```python
from build123d import *

# Parameters (mm, degrees)
SKETCH1_R           = 1.5
BOSS_EXTRUDE1_DEPTH = 8
SKETCH2_R           = 4
SKETCH2_R_2         = 1.5
BOSS_EXTRUDE2_DEPTH = 2
SKETCH4_R           = 4
SKETCH4_R_2         = 2.75
BOSS_EXTRUDE3_DEPTH = 2.5
CUT_EXTRUDE1_DEPTH  = 3
BOSS_EXTRUDE4_DEPTH = 5
BOSS_EXTRUDE5_DEPTH = 2.5
BOSS_EXTRUDE6_DEPTH = 13
BOSS_EXTRUDE7_DEPTH = 8
CUT_EXTRUDE4_START  = -5
SKETCH16_R          = 35.00000000000001
SKETCH16_R_2        = 33.50186054017001
CUT_EXTRUDE4_DEPTH  = 5
FILLET2_R           = 5
SKETCH6_R           = 1.500000000000004
CUT_EXTRUDE5_DEPTH  = 72.01408318918156
SKETCH6_8_R         = 1.500000000000004
CUT_EXTRUDE6_DEPTH  = 3
SKETCH17_R          = 3.999999999999999
SKETCH17_R_2        = 1.500000000000004
BOSS_EXTRUDE8_DEPTH = 2
SKETCH18_R          = 4.000000000000003
SKETCH18_R_2        = 2.7500000000000018
BOSS_EXTRUDE9_DEPTH = 2.5


with BuildPart() as part:
    # Sketch1 → Boss-Extrude1 (new body)
    with BuildSketch(Plane(origin=(0, 0, 0), x_dir=(1, 0, 0), z_dir=(0, 1, 0))):
        with BuildLine():
            Line((-7.5, 36.50000000000001), (-43, 36.5))
            Line((-43, 36.5), (-43, 32.5))
            Line((-43, 32.5), (-17.500000000000068, 32.49999999999999))
            ThreePointArc((-17.500000000000068, 32.49999999999999), (-10.428932188134521, 29.571067811865472), (-7.499999999999997, 22.499999999999922))
            Line((-7.499999999999997, 22.499999999999922), (-7.5, 0))
            ThreePointArc((-7.5, 0), (-1.38e-15, -7.5), (7.5, 0))
            Line((7.5, 0), (7.5, 40))
            ThreePointArc((7.5, 40), (5.303300858899107, 45.30330085889911), (1.7e-16, 47.5))
            Line((1.7e-16, 47.5), (-19, 47.5))
            Line((-19, 47.5), (-19, 42.5))
            Line((-19, 42.5), (-7.5, 42.5))
            Line((-7.5, 42.5), (-7.5, 36.50000000000001))
        make_face()
        with Locations(Location((0, 0, 0), (0, 0, 270))):
            Circle(SKETCH1_R, mode=Mode.SUBTRACT)
        with BuildLine():
            ThreePointArc((-3.822328563123411, 25.208378945159915), (-4.975312131849936, 23.47239594738329), (-3.2806101420555054, 22.2595508442844))
            ThreePointArc((-3.2806101420555054, 22.2595508442844), (-0.0667184196164731, 22.499901229693076), (3.1485421826830366, 22.278615056087435))
            ThreePointArc((3.1485421826830366, 22.278615056087435), (4.959579589511544, 23.370856111085427), (3.8935926199376825, 25.19747013486111))
            ThreePointArc((3.8935926199376825, 25.19747013486111), (0.03604708010283943, 25.496495157085157), (-3.822328563123411, 25.208378945159915))
        make_face(mode=Mode.SUBTRACT)
    extrude(amount=BOSS_EXTRUDE1_DEPTH)

    # Sketch2 → Boss-Extrude2 (add)
    with BuildSketch(Plane(origin=(0, 8, 0), x_dir=(1, 0, 0), z_dir=(0, 1, 0))):
        with Locations(Location((0, 0, 0), (0, 0, 270))):
            Circle(SKETCH2_R)
        with Locations(Location((0, 0, 0), (0, 0, 270))):
            Circle(SKETCH2_R_2, mode=Mode.SUBTRACT)
    extrude(amount=BOSS_EXTRUDE2_DEPTH)

    # Sketch4 → Boss-Extrude3 (add)
    with BuildSketch(Plane(origin=(0, 10, 0), x_dir=(1, 0, 0), z_dir=(0, 1, 0))):
        with Locations(Location((0, 0, 0), (0, 0, 270))):
            Circle(SKETCH4_R)
        with Locations(Location((0, 0, 0), (0, 0, 270))):
            Circle(SKETCH4_R_2, mode=Mode.SUBTRACT)
    extrude(amount=BOSS_EXTRUDE3_DEPTH)

    # Sketch5 → Cut-Extrude1 (cut)
    with BuildSketch(Plane(origin=(0, 8, 0), x_dir=(1, 0, 0), z_dir=(0, 1, 0))):
        with BuildLine():
            ThreePointArc((-3.901041666666667, 26.46402036567631), (-6.220600224508779, 23.342378474500862), (-3.098958333333334, 21.022819916658754))
            ThreePointArc((-3.098958333333334, 21.022819916658754), (1.3e-15, 21.250000000000004), (3.098958333333334, 21.022819916658754))
            ThreePointArc((3.098958333333334, 21.022819916658754), (6.220600224508775, 23.342378474500865), (3.901041666666667, 26.46402036567631))
            ThreePointArc((3.901041666666667, 26.46402036567631), (1.64e-15, 26.749999999999996), (-3.901041666666667, 26.46402036567631))
        make_face()
    extrude(amount=-CUT_EXTRUDE1_DEPTH, mode=Mode.SUBTRACT)

    # Sketch11 → Boss-Extrude4 (add)
    with BuildSketch(Plane(origin=(0, 8, 0), x_dir=(1, 0, 0), z_dir=(0, 1, 0))):
        with BuildLine():
            Line((-19, 42.5), (-7.5, 42.5))
            Line((-7.5, 42.5), (-7.5, 36.50000000000001))
            Line((-7.5, 36.50000000000001), (-43, 36.5))
            Line((-43, 36.5), (-43, 32.5))
            Line((-43, 32.5), (-17.500000000000064, 32.49999999999999))
            ThreePointArc((-17.500000000000064, 32.49999999999999), (-15.859503936382302, 32.36452090398995), (-14.263458457505935, 31.961754533050943))
            ThreePointArc((-14.263458457505937, 31.961754533050936), (-3.5600570438609966, 34.81847202053036), (7.5, 34.18698582794336))
            Line((7.5, 34.18698582794336), (7.5, 40))
            ThreePointArc((7.5, 40), (5.303300858899107, 45.30330085889911), (1.3e-16, 47.5))
            Line((9.2e-16, 47.5), (-19, 47.5))
            Line((-19, 47.5), (-19, 42.5))
        make_face()
    extrude(amount=BOSS_EXTRUDE4_DEPTH)

    # Sketch12 → Boss-Extrude5 (add)
    with BuildSketch(Plane.XY.offset(-32.499999999999986)):
        Polygon((-43.00000000000001, 0), (-17.500000000000078, 0), (-17.500000000000085, 13.000000000000002), (-43.00000000000001, 13.000000000000002), align=None)
    extrude(amount=BOSS_EXTRUDE5_DEPTH)

    # Sketch14 → Boss-Extrude6 (add)
    with BuildSketch(Plane(origin=(0, 0, 0), x_dir=(1, 0, 0), z_dir=(0, 1, 0))):
        with BuildLine():
            Line((-17.500000000000068, 30.310889132455326), (-17.500000000000075, 32.49999999999999))
            ThreePointArc((-17.500000000000075, 32.49999999999999), (-15.859503936382307, 32.364520903989956), (-14.263458457505932, 31.961754533050946))
            ThreePointArc((-14.263458457505932, 31.961754533050946), (-15.903165170435354, 31.178347255136085), (-17.500000000000068, 30.310889132455326))
        make_face()
    extrude(amount=BOSS_EXTRUDE6_DEPTH)

    # Sketch15 → Boss-Extrude7 (add)
    with BuildSketch(Plane(origin=(0, 0, 0), x_dir=(1, 0, 0), z_dir=(0, 1, 0))):
        with BuildLine():
            Line((-17.500000000000075, 29.99999999999999), (-17.500000000000068, 30.310889132455326))
            ThreePointArc((-17.500000000000068, 30.310889132455326), (-15.90316517043534, 31.178347255136092), (-14.263458457505916, 31.961754533050954))
            ThreePointArc((-14.263458457505916, 31.961754533050954), (-12.477821634213894, 31.14741143130302), (-10.8856217223385, 29.99999999999999))
            Line((-10.8856217223385, 29.99999999999999), (-17.500000000000075, 29.99999999999999))
        make_face()
    extrude(amount=BOSS_EXTRUDE7_DEPTH)

    # Sketch16 → Cut-Extrude4 (cut)
    with BuildSketch(Plane(origin=(0, 13.000000000000002, 0), x_dir=(1, 0, 0), z_dir=(0, 1, 0)).offset(CUT_EXTRUDE4_START)):
        Circle(SKETCH16_R)
        Circle(SKETCH16_R_2, mode=Mode.SUBTRACT)
    extrude(amount=CUT_EXTRUDE4_DEPTH, mode=Mode.SUBTRACT)

    # Fillet2
    fillet2_edges = [part.edges().sort_by_distance(p)[0] for p in [
        (-5.664903014694951, 8, -34.5385129071027),
    ]]
    fillet(fillet2_edges, radius=FILLET2_R - 0.0001)  # a hair under: the kernel refuses the full size

    # Sketch6 → Cut-Extrude5 (cut, through all)
    with BuildSketch(Plane(origin=(0, 0, -47.5), x_dir=(-1, 0, 0), z_dir=(0, 0, -1))):
        with BuildLine():
            ThreePointArc((12.740543617655444, 9.78125), (11.475329858832474, 11.483963758822968), (9.772616100009506, 10.21875))
            ThreePointArc((9.772616100009506, 10.21875), (9.50000000000001, 6.5000000000000036), (9.772616100009508, 2.7812499999999982))
            ThreePointArc((9.772616100009508, 2.7812499999999982), (11.475329858832469, 1.5160362411770363), (12.740543617655444, 3.218749999999997))
            ThreePointArc((12.740543617655444, 3.218749999999997), (12.500000000000004, 6.500000000000003), (12.740543617655444, 9.78125))
        make_face()
        with Locations(Location((35, 6.5, 0), (0, 0, 180))):
            Circle(SKETCH6_R)
    extrude(amount=-CUT_EXTRUDE5_DEPTH, mode=Mode.SUBTRACT)

    # Sketch6<8> → Cut-Extrude6 (cut)
    # profile 1 of 2: a face of its own
    with BuildSketch(Plane(origin=(0, 0, -47.5), x_dir=(-1, 0, 0), z_dir=(0, 0, -1))):
        with Locations(Location((35, 6.5, 0), (0, 0, 180))):
            Circle(SKETCH6_8_R)
    # profile 2 of 2: a face of its own
    with BuildSketch(Plane(origin=(0, 0, -47.5), x_dir=(-1, 0, 0), z_dir=(0, 0, -1))):
        with BuildLine():
            ThreePointArc((13.977180083341253, 9.598958333333332), (11.65762152549914, 12.720600224508777), (8.535979634323695, 10.401041666666664))
            ThreePointArc((8.535979634323695, 10.401041666666664), (8.250000000000007, 6.5000000000000036), (8.535979634323692, 2.5989583333333335))
            ThreePointArc((8.535979634323692, 2.5989583333333335), (11.657621525499136, 0.27939977549122075), (13.97718008334125, 3.401041666666666))
            ThreePointArc((13.97718008334125, 3.401041666666666), (13.750000000000004, 6.500000000000003), (13.977180083341253, 9.598958333333332))
        make_face()
        with BuildLine():
            ThreePointArc((12.740543617655444, 9.78125), (11.475329858832474, 11.483963758822968), (9.772616100009506, 10.21875))
            ThreePointArc((9.772616100009506, 10.21875), (9.50000000000001, 6.5000000000000036), (9.772616100009508, 2.7812499999999982))
            ThreePointArc((9.772616100009508, 2.7812499999999982), (11.475329858832469, 1.5160362411770363), (12.740543617655444, 3.218749999999997))
            ThreePointArc((12.740543617655444, 3.218749999999997), (12.500000000000004, 6.500000000000003), (12.740543617655444, 9.78125))
        make_face(mode=Mode.SUBTRACT)
    extrude(amount=-CUT_EXTRUDE6_DEPTH, mode=Mode.SUBTRACT)

    # Sketch17 → Boss-Extrude8 (add)
    with BuildSketch(Plane.XY.offset(-29.99999999999999)):
        with Locations((-35, 6.5)):
            Circle(SKETCH17_R)
        with Locations((-35, 6.5)):
            Circle(SKETCH17_R_2, mode=Mode.SUBTRACT)
    extrude(amount=BOSS_EXTRUDE8_DEPTH)

    # Sketch18 → Boss-Extrude9 (add)
    with BuildSketch(Plane.XY.offset(-27.99999999999999)):
        with Locations((-35, 6.5)):
            Circle(SKETCH18_R)
        with Locations((-35, 6.5)):
            Circle(SKETCH18_R_2, mode=Mode.SUBTRACT)
    extrude(amount=BOSS_EXTRUDE9_DEPTH)


solid = part.part
```
Geometry check sheet. Reference: the model listing, model coordinates, mm. A direction names the side the tool comes from. Coordinates: 2 decimals unless noted, no trailing zeros. Loops run counter-clockwise (first coordinate to the right, second up) from the corner with the lowest first, then second, coordinate; pieces in that order, holes last.
Item 1: Sectioned sample at C-C, the plane z = -13. Record the boundary of the cut face in (x, y).
Item 2: Access from +Z, -Z, +X, -X, +Y, -Y to the whole of each face (thin tool, end or side, straight path). Record for faces 1 (the face through (-4.98, 2.46, -23.5)), 2 (the face through (-9.5, 6.6, -32.6)), 3 (the face through (-13.75, 6.46, -46.02)), 4 (the face through (-3.905, 10.218, -0.867)), 5 (the face through (-3, 12.5, -1)).
Item 3: Release check for a two-part mould opening along X. For faces 6 (the face through (-7.5, 4, -11)), 7 (the face through (-11.51, 11.48, -34.53)), 8 (the face through (-9.5, 6.6, -43.5)), 9 (the face through (-32, 7, -25.5)) record: released by +X, released by -X, zero draft, split by the parting line, or undercut.
Item 4: Sectioned sample at A-A, the plane x = -35. Record the boundary of the cut face in (y, z).
Item 5: Go/stop test with flat-tipped pins: pin 1 Ø1.8 at (y, z) = (4.5, -38.5) entering from -X; pin 2 Ø6.5 at (x, y) = (-35, 6.5) entering from -Z; pin 3 Ø5 at (x, z) = (-2, -3) entering from +Y. Record where each tip stops, or that it passes through.
Item 6: Sectioned sample at B-B, the plane y = 6.5. Count the separate pieces of the cut face and the enclosed holes in it, then the cut area to 3 significant figures.
Item 7: Thickness scan on line 1 (X direction, y = 6.5, z = -34.25); line 2 (Z direction, x = -16, y = 7.5); line 3 (Z direction, x = 1, y = 12). Record the ranges inside material, lowest first.
Check result:
1. outline: (-7.5, 0) - (7.5, 0) - (7.5, 8) - (-7.5, 8) - close
2. face 1: +Y, -Y
2. face 2: +Z, -Z
2. face 3: -Z
2. face 4: +Y
2. face 5: +Z, +X, -X, +Y
3. face 6: released by -X
3. face 7: undercut
3. face 8: undercut
3. face 9: zero draft
4. outline: (0, -36.5) - (5, -36.5) - (5, -28) - (3.75, -28) - (3.75, -25.5) - (2.5, -25.5) - (2.5, -30) - (0, -30) - close; (8, -36.5) - (13, -36.5) - (13, -30) - (10.5, -30) - (10.5, -25.5) - (9.25, -25.5) - (9.25, -28) - (8, -28) - close
5. pin 1: stops at x = -7.5
5. pin 2: stops at z = -36.5
5. pin 3: stops at y = 12.5
6. separate pieces: 4
6. enclosed holes: 2
6. area: 969 mm2
7. line 1: x = -43 to -36.5, -33.5 to -12.5, -9.5 to 7.5
7. line 2: z = -47.5 to -42.5, -36.5 to -30
7. line 3: z = -47.43 to -34.88, -3.87 to -2.56, 2.56 to 3.87
